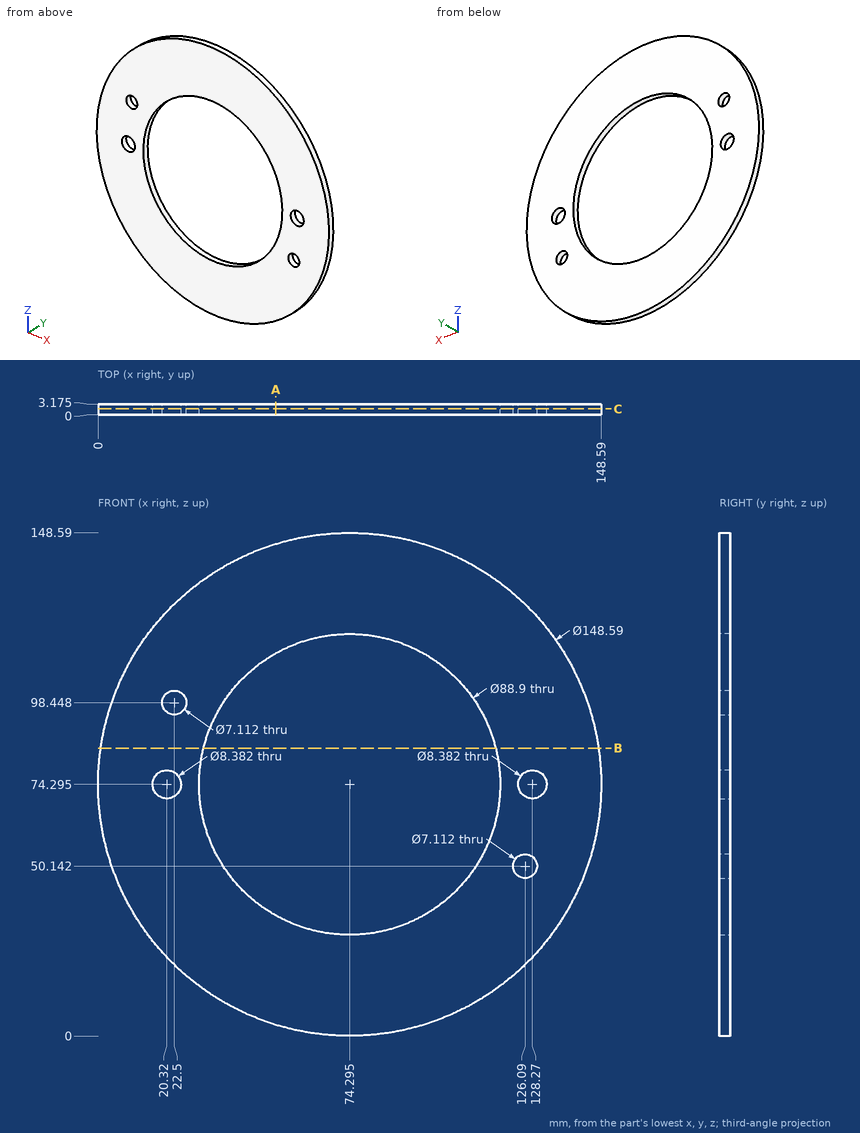
Drawing for the job (mm, zero at the part's lowest x, y, z). Coordinates: 2 decimals unless noted, no trailing zeros. Write each loop counter-clockwise with the first axis right and the second up, starting at its lowest first coordinate (ties: lowest second). Pieces come first, ordered by that corner, then holes. Notation, with made-up numbers: (-10, 70) -> (-2, 70) arc R30 cw to (-2, 97) -> close; hole circle Ø7 at (-25, -23.75). An arc over 180 degrees is marked (long way). One line per item, written item: value. Start each with the question number.
1) Flat gauge pins, fed straight in: pin 1 Ø1.5 at (x, y) = (100, 0.5) entering from +Z; pin 2 Ø1 at (y, z) = (1.5, 87.5) entering from +X (1 decimal). Where does each tip first touch, or does it go through?
2) Slice it at C-C on y = 1.75. Count the separate pieces of the cut face and the enclosed holes in it, then the cut area to 3 significant figures.
3) Probe probe 1 along Z at (x, y) = (74, 0.4) (1 decimal); probe 2 along Z at (x, y) = (94, 0.2); probe 3 along X at (y, z) = (2, 55.5) (1 decimal). List the from-to ranges inside material, lowest first.
4) Slice it at A-A on x = 52.5. Write the cut outline in (y, z) (1 decimal).
5) Slice it at B-B on z = 85. Write the cut outline in (x, y) (1 decimal).
Answers follow:
1. pin 1: z = 144.27
1. pin 2: x = 147.5
2. separate pieces: 1
2. enclosed holes: 5
2. area: 10,900 mm2
3. probe 1: 0 to 29.8, 118.7 to 148.6
3. probe 2: 2.66 to 34.45, 114.14 to 145.93
3. probe 3: 2.4 to 34, 114.6 to 146.2
4. outline: (0, 3.3) -> (3.2, 3.3) -> (3.2, 35.6) -> (0, 35.6) -> close; (0, 113) -> (3.2, 113) -> (3.2, 145.3) -> (0, 145.3) -> close
5. outline: (0.8, 0) -> (31.2, 0) -> (31.2, 3.2) -> (0.8, 3.2) -> close; (117.4, 0) -> (147.8, 0) -> (147.8, 3.2) -> (117.4, 3.2) -> close
